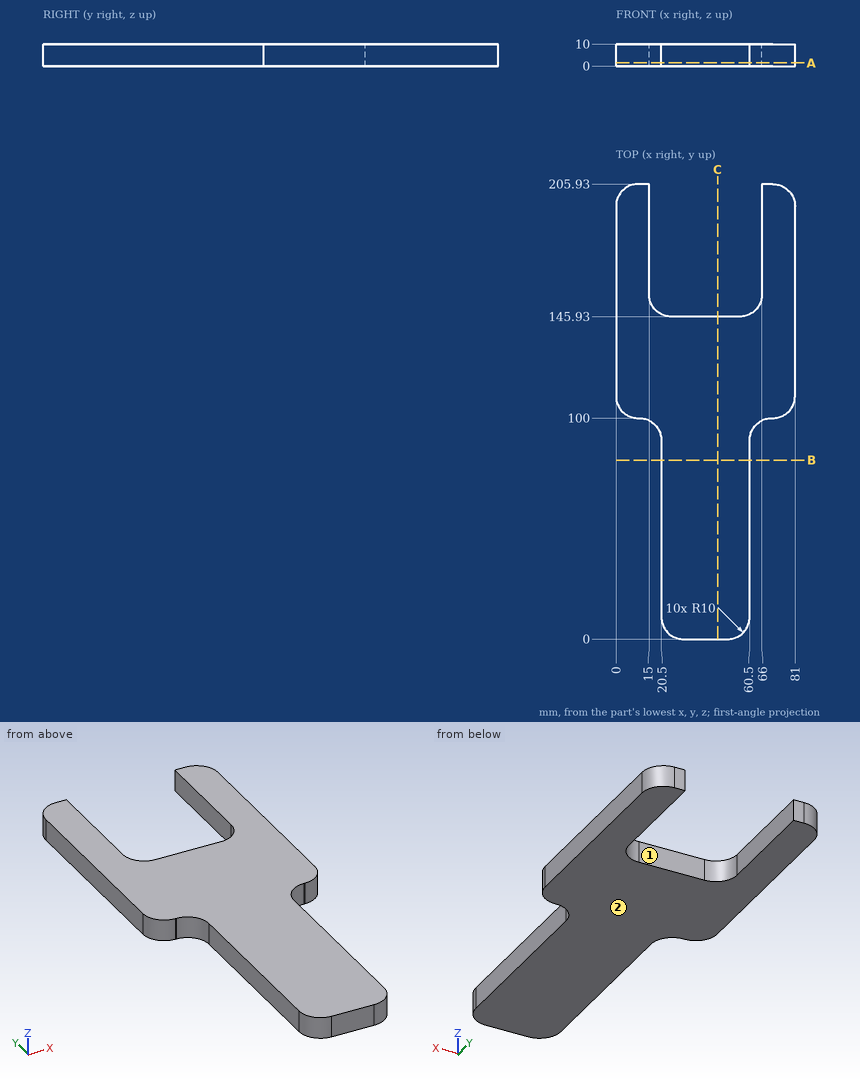
Job drawing, mm, ordinate dimensions from the low corner. One solid piece. A direction names the side the tool comes from. Round coordinates to 2 decimals unless told otherwise and drop trailing zeros. Order: outer loops, then holes, each group sorted by start corner. A loop starts at its lowest first (then second) coordinate and runs counter-clockwise, first axis right, second up. Notation, with made-up numbers: (83.25, -1) - (122.25, -1) arc R20 cw to (122.25, 3) - close; hole circle Ø8 at (-24, -21). An arc over 180 degrees is marked (long way). Use CSV: the item, a comma, the result in double quotes. Start each with the question number.
1) Tool access for the marked faces 1 and 2: list every direction of +Z, -Z, +X, -X, +Y, -Y with a clear straight run to the whole face (end or side of a thin tool).
2) Wall check: L1, parallel to X at y = 169.5, z = 3.75; L2, parallel to Y at x = 34.5, z = 6.75; L3, parallel to X at y = 55, z = 2.25. Give the ranges that are in metal, low to high. Write a range as [from, to].
3) Saw through at A-A (z = 1.5). List the corners of the cut face in (x, y).
4) Pin check, flat tips, straight feed: pin 1 Ø5 at (x, z) = (38, 3) entering from +Y; pin 2 Ø5 at (y, z) = (52.5, 4) entering from -X; pin 3 Ø4 at (x, z) = (14.5, 2.5) entering from -Y. Stop position of each tip, or through.
5) Saw through at B-B (y = 81). List the corners of the cut face in (x, z).
6) Saw through at C-C (x = 46). List the corners of the cut face in (y, z).
Values follow:
1,face 1,"+Z, -Z, +Y"
1,face 2,"-Z, +X, -X, +Y, -Y"
2,L1,"x = [0, 15], [66, 81]"
2,L2,"y = [0, 145.93]"
2,L3,"x = [20.5, 60.5]"
3,outline,"(0, 110) arc R10 ccw to (10, 100) - (10.5, 100) arc R10 cw to (20.5, 90) - (20.5, 10) arc R10 ccw to (30.5, 0) - (50.5, 0) arc R10 ccw to (60.5, 10) - (60.5, 90) arc R10 cw to (70.5, 100) - (71, 100) arc R10 ccw to (81, 110) - (81, 195.93) arc R10 ccw to (71, 205.93) - (66, 205.93) - (66, 155.93) arc R10 cw to (56, 145.93) - (25, 145.93) arc R10 cw to (15, 155.93) - (15, 205.93) - (10, 205.93) arc R10 ccw to (0, 195.93) - close"
4,pin 1,"stops at y = 145.93"
4,pin 2,"stops at x = 20.5"
4,pin 3,"stops at y = 98"
5,outline,"(20.5, 0) - (60.5, 0) - (60.5, 10) - (20.5, 10) - close"
6,outline,"(0, 0) - (145.93, 0) - (145.93, 10) - (0, 10) - close"
